Job drawing, mm, ordinate dimensions from the low corner. One solid piece. A direction names the side the tool comes from. Give positions to 0.01 mm unless a question says otherwise; leave off trailing zeros. Loops run counter-clockwise (first coordinate to the right, second up) from the corner with the lowest first, then second, coordinate; pieces in that order, holes last. Notation, with made-up numbers: M 81,11.5 L 85,11.5 A19 ccw 85,26.5 Z; hole C 23.25,-22.75 d4. An arc over 180 degrees is marked long. One line per question, with ' | ' between items.
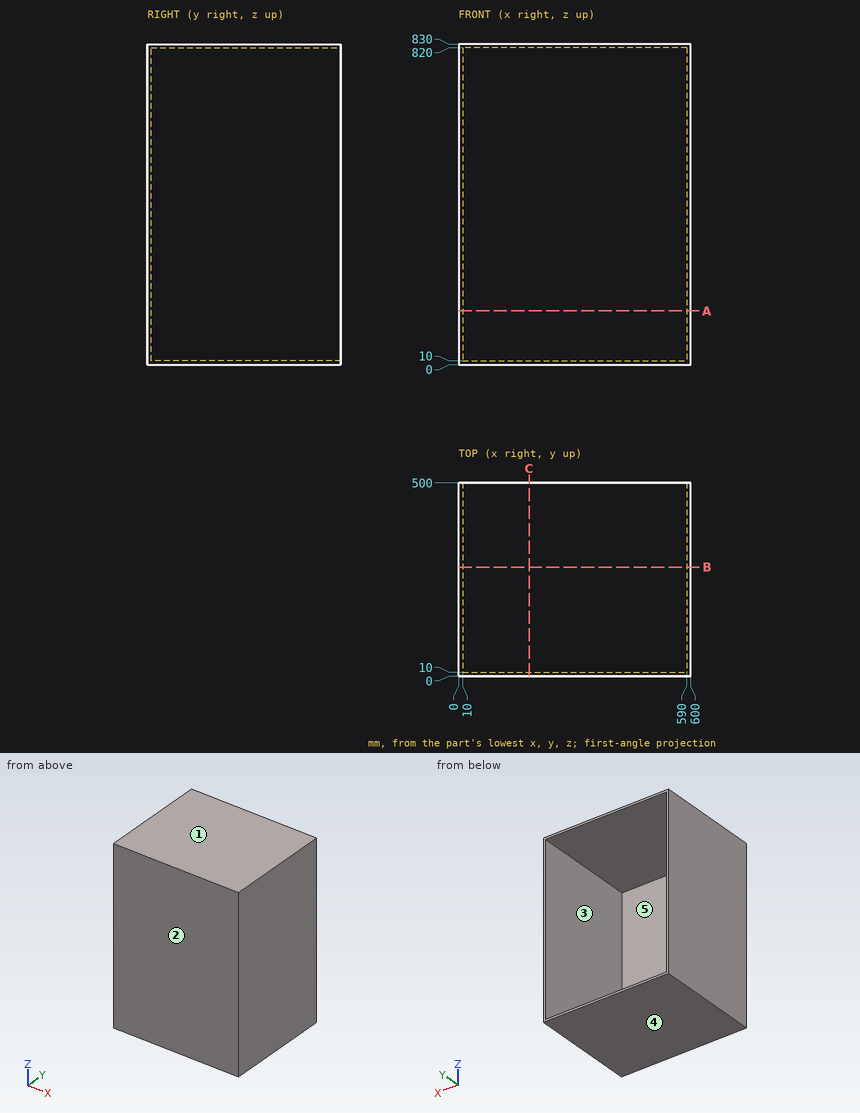
Item 1: Saw through at B-B on y = 282. Give the cut face in (x, z), and give its area (3 significant figures).
Conclusion:
outline: M 0,0 L 600,0 L 600,830 L 0,830 Z; hole M 10,10 L 590,10 L 590,820 L 10,820 Z | area: 28,200 mm²
Item 2: Drop a flat-ended pin along its axis: P1, Ø8, axis at x = 386, z = 638.5, coming from the +Y side. Give the stop position or say it passes through.
Conclusion:
P1: y = 10
Item 3: Saw through at A-A on z = 139.5. Give the cut face in (x, y), and give its area (3 significant figures).
Conclusion:
outline: M 0,0 L 600,0 L 600,500 L 590,500 L 590,10 L 10,10 L 10,500 L 0,500 Z | area: 15,800 mm²
Item 4: 3-axis set-ups, long thin cutter, end or side, ignore diameter. For the marked faces 4 and 5: which of +Z, -Z, +X, -X, +Y, -Y reach the whole face in a straight line?
Conclusion:
face 4: -Z, +X, -X, +Y, -Y | face 5: +Y
Item 5: Mould opens along Z. For the marked faces 1, 2 and 3 say: pulls with the +Z half, pulls with the -Z half, needs draft (parallel to the pull), parting line crosses it, or undercut.
Conclusion:
face 1: pulls with the +Z half | face 2: needs draft | face 3: undercut
Item 6: Drill centre lines: line 1 along X through (y, z) = (456.5, 592); line 2 along Z through (x, y) = (206, 135); line 3 along Y through (x, z) = (470.5, 659.5). Where is each one in solid material? Low to high. Write a range as [from, to].
Conclusion:
line 1: [0, 10], [590, 600] | line 2: [0, 10], [820, 830] | line 3: [0, 10]
Item 7: Saw through at C-C on x = 182. Give the cut face in (y, z).
Conclusion:
outline: M 0,0 L 500,0 L 500,10 L 10,10 L 10,820 L 500,820 L 500,830 L 0,830 Z
